```python
from build123d import *

# Parameters (mm, degrees)
SKETCH_R      = 14.25
PAD_DEPTH     = 8
SKETCH001_R   = 15.9
PAD001_DEPTH  = 0.3
SKETCH002_R   = 13.25
PAD002_DEPTH  = 3.5
SKETCH003_R   = 10.5
SKETCH003_R_2 = 8.5
PAD003_DEPTH  = 2.5
SKETCH004_R   = 6.9
POCKET_DEPTH  = 11.801
FILLET_R      = 1
FILLET001_R   = 1


with BuildPart() as part:
    # Sketch → Pad (new body)
    with BuildSketch(Plane.XY):
        Circle(SKETCH_R)
    extrude(amount=PAD_DEPTH)

    # Sketch001 (on Face3 of Pad) → Pad001 (join)
    with BuildSketch(Plane.XY.offset(8)):
        Circle(SKETCH001_R)
    extrude(amount=PAD001_DEPTH)

    # Sketch002 (on Face3 of Pad001) → Pad002 (join)
    with BuildSketch(Plane.XY.offset(8.3)):
        Circle(SKETCH002_R)
    extrude(amount=PAD002_DEPTH)

    # Sketch003 (on Face7 of Pad002) → Pad003 (join)
    with BuildSketch(Plane.XY.offset(11.8)):
        Circle(SKETCH003_R)
        Circle(SKETCH003_R_2, mode=Mode.SUBTRACT)
    extrude(amount=PAD003_DEPTH)

    # Sketch004 (on Face11 of Pad003) → Pocket (cut, through all)
    with BuildSketch(Plane.XY.offset(11.8)):
        Circle(SKETCH004_R)
    extrude(amount=-POCKET_DEPTH, mode=Mode.SUBTRACT)

    # Fillet
    fillet_edges = [part.edges().sort_by_distance(p)[0] for p in [
        (-14.25, 0, 0),
    ]]
    fillet(fillet_edges, radius=FILLET_R)

    # Fillet001
    fillet001_edges = [part.edges().sort_by_distance(p)[0] for p in [
        (-6.9, 0, 0),
    ]]
    fillet(fillet001_edges, radius=FILLET001_R)


solid = part.part
```
The listing builds one solid part. Answer for the finished solid, in the listing's coordinates (mm). A direction names the side the tool comes from. Round coordinates to 2 decimals unless told otherwise and drop trailing zeros. Write each loop counter-clockwise with the first axis right and the second up, starting at its lowest first coordinate (ties: lowest second). Pieces come first, ordered by that corner, then holes. Notation, with made-up numbers: (74.25, 15) -> (110.25, 15) arc R16 cw to (110.25, 24) -> close; hole circle Ø4 at (8, 60.5). An arc over 180 degrees is marked (long way). Use CSV: the item, a comma, the result in double quotes. Start each with the question number.
(1) Section A-A on y = 0 is taken. Give the vertices of the cut face in (x, z), then the cut area to 3 significant figures.
(2) Which of the six approach directions +Z, -Z, +X, -X, +Y, -Y give full straight-line access (tool end or side, diameter ignored) to faces 1 (the face through (13.163, -5.458, 4.451)), 2 (the face through (-1, 7, 11.8)), 3 (the face through (9, 0, 14.3))?
(3) Consider L1, parallel to Y at x = 0, z = 13.15; L2, parallel to Y at x = 0, z = 4.5; L3, parallel to Z at x = -6.5, y = 14. Determine where each line is inside the solid, lowest interval first. Write a range as from..to.
(4) The mould has two halves that part along X. Classify faces 4 (the face through (10, 3.2, 13)), 5 (the face through (4.57, 7.167, 13.032)), 6 (the face through (-6, 12, 8.3)): released by +X, released by -X, zero draft, split by the parting line, or undercut.
(5) Each of these flat-tipped pins is pushed along its axis until it touches: pin 1 (15.5 mm diameter, centred on x = 0, y = 0, fed in from -Z); pin 2 (2 mm diameter, centred on y = -9, z = 5, fed in from -X); pin 3 (3 mm diameter, centred on y = -1.5, z = 4, fed in from -X). Where does it stop, or does it pass through?
(6) Section C-C on z = 7.5 is taken. Give the vertices of the cut face in (x, y).
A:
1,outline,"(-15.9, 8) -> (-14.25, 8) -> (-14.25, 1) arc R1 ccw to (-13.25, 0) -> (-7.9, 0) arc R1 ccw to (-6.9, 1) -> (-6.9, 11.8) -> (-8.5, 11.8) -> (-8.5, 14.3) -> (-10.5, 14.3) -> (-10.5, 11.8) -> (-13.25, 11.8) -> (-13.25, 8.3) -> (-15.9, 8.3) -> close; (6.9, 1) arc R1 ccw to (7.9, 0) -> (13.25, 0) arc R1 ccw to (14.25, 1) -> (14.25, 8) -> (15.9, 8) -> (15.9, 8.3) -> (13.25, 8.3) -> (13.25, 11.8) -> (10.5, 11.8) -> (10.5, 14.3) -> (8.5, 14.3) -> (8.5, 11.8) -> (6.9, 11.8) -> close"
1,area,"177 mm²"
2,face 1,"-Z"
2,face 2,"+Z"
2,face 3,"+Z, +X, -X, +Y, -Y"
3,L1,"y = -10.5..-8.5, 8.5..10.5"
3,L2,"y = -14.25..-6.9, 6.9..14.25"
3,L3,"z = 8..8.3"
4,face 4,"split by the parting line"
4,face 5,"undercut"
4,face 6,"zero draft"
5,pin 1,"stops at z = 0.01"
5,pin 2,"stops at x = -11.79"
5,pin 3,"stops at x = -14.25"
6,outline,"circle Ø28.5 at (0, 0); hole circle Ø13.8 at (0, 0)"
